Input: part model. Units: mm. Frame: model coordinates. Coordinates: 2 decimals unless noted, no trailing zeros. Write each loop counter-clockwise with the first axis right and the second up, starting at its lowest first coordinate (ties: lowest second). Pieces come first, ordered by that corner, then holes. Notation, with made-up numbers: (25.5, 31.25) - (30.5, 31.25) arc R18 ccw to (30.5, 45.25) - close; hole circle Ø9 at (5, 71.25). An arc over 180 degrees is marked (long way). Use a Markdown table: item, result. Add a question column.
Q1. Section query D-D (y = -0.75). Return the cut outline in (x, z).
Q2. Pin query (flat end, axial travel): P1, Ø1, axis at x = -9.5, z = -4, coming from the -Y side; P2, Ø2, axis at y = 5.5, z = -4, coming from the +X side; P3, Ø1.5, axis at x = 1.5, z = -3, coming from the +Y side. Return the tip coordinate at first contact, or that it passes through.
Q3. Material intervals for probe 1 along Z at (x, y) = (-10, 1); probe 2 along Y at (x, z) = (28, -3.25); probe 3 along X at (y, z) = (6, 1.75), sorted ascending. Write a range as from..to.
Q4. Section query B-B (x = -30). Return the cut outline in (y, z), then the cut area to 3 significant figures.
Q5. Section query A-A (z = -2.25). Return the cut outline in (x, y).
Autodesk Fusion 360 part; units mm, degrees
sketch "Sketch1" plane through (0, 0, 0) normal (0, 0, 1) x (1, 0, 0) in component "Cover"
  line L0 (34, 8.25) -> (-34, 8.25)
  line L1 (-34, 8.25) -> (-34, -8.25)
  line L2 (-34, -8.25) -> (34, -8.25)
  line L3 (34, -8.25) -> (34, 8.25)
  line L4 (34, 8.25) -> (-34, -8.25) construction
  line L5 (-34, 8.25) -> (34, -8.25) construction
  line L6 (-32.5, -6.75) -> (32.5, -6.75) construction
  line L7 (32.5, -6.75) -> (32.5, 6.75) construction
  line L8 (32.5, 6.75) -> (-32.5, 6.75)
  line L9 (-32.5, 6.75) -> (-32.5, -6.75) construction
  line L10 (32.5, 4.25) -> (24.6, 4.25)
  line L11 (24.6, 4.25) -> (24.6, 6.75)
  line L12 (24.6, 6.75) -> (32.5, 6.75)
  line L13 (32.5, 6.75) -> (32.5, 4.25)
  line L14 (22.9833, 6.75) -> (22.9833, 4.25)
  line L15 (15.0833, 4.25) -> (15.0833, 6.75)
  line L16 (22.9833, 4.25) -> (15.0833, 4.25)
  line L17 (15.0833, 6.75) -> (22.9833, 6.75)
  line L18 (13.4667, 6.75) -> (13.4667, 4.25)
  line L19 (5.5667, 4.25) -> (5.5667, 6.75)
  line L20 (13.4667, 4.25) -> (5.5667, 4.25)
  line L21 (5.5667, 6.75) -> (13.4667, 6.75)
  line L22 (3.95, 6.75) -> (3.95, 4.25)
  line L23 (-3.95, 4.25) -> (-3.95, 6.75)
  line L24 (3.95, 4.25) -> (-3.95, 4.25)
  line L25 (-3.95, 6.75) -> (3.95, 6.75)
  line L26 (-5.5667, 6.75) -> (-5.5667, 4.25)
  line L27 (-13.4667, 4.25) -> (-13.4667, 6.75)
  line L28 (-5.5667, 4.25) -> (-13.4667, 4.25)
  line L29 (-13.4667, 6.75) -> (-5.5667, 6.75)
  line L30 (-15.0833, 6.75) -> (-15.0833, 4.25)
  line L31 (-22.9833, 4.25) -> (-22.9833, 6.75)
  line L32 (-15.0833, 4.25) -> (-22.9833, 4.25)
  line L33 (-22.9833, 6.75) -> (-15.0833, 6.75)
  line L34 (-24.6, 6.75) -> (-24.6, 4.25)
  line L35 (-32.5, 4.25) -> (-32.5, 6.75)
  line L36 (-24.6, 4.25) -> (-32.5, 4.25)
  line L37 (-32.5, 6.75) -> (-24.6, 6.75)
  line L38 (-34, -8.25) -> (-36, -8.25)
  line L39 (-36, -8.25) -> (-36, 8.25)
  line L40 (-36, 8.25) -> (-34, 8.25)
  line L41 (-34, 8.25) -> (-34, -8.25)
  line L42 (34, -8.25) -> (36, -8.25)
  line L43 (36, -8.25) -> (36, 8.25)
  line L44 (36, 8.25) -> (34, 8.25)
  line L45 (34, 8.25) -> (34, -8.25)
  dimension "d39" = 68
  dimension "d40" = 16.5
  dimension "d42" = 7.9
  dimension "d43" = 2.5
  dimension "d46" = -57.1
  dimension "d47" = 0
  dimension "d52" = 2
  dimension "d53" = 2
extrude "Extrude1" add sketch "Sketch1" along normal blind 2 contours L0 L1 L2 L3 L41 L45 | L3 L42 L43 L44 L45 | L1 L38 L39 L40 L41 | L8 L10 L11 L12 L13 | L8 L34 L35 L36 L37 | L8 L30 L31 L32 L33 | L8 L26 L27 L28 L29 | L8 L22 L23 L24 L25 | L8 L18 L19 L20 L21 | L8 L14 L15 L16 L17 in component "Cover"
extrude "Extrude3" add sketch "Sketch1" against normal blind 5 contours L8 L10 L11 L12 L13 | L8 L34 L35 L36 L37 | L8 L30 L31 L32 L33 | L8 L26 L27 L28 L29 | L8 L22 L23 L24 L25 | L8 L18 L19 L20 L21 | L8 L14 L15 L16 L17 in component "Cover"
fillet "Fillet1" radius 3 7 edges at (28.55, 4.25, 0) (19.0333, 4.25, 0) (9.5167, 4.25, 0) (0, 4.25, 0) (-9.5167, 4.25, 0) (-19.0333, 4.25, 0) (-28.55, 4.25, 0) in component "Cover"
chamfer "Chamfer2" distance 0.4 angle 45 1 faces at (1.3167, -3.25, 2) in component "Cover"
component "Cover" placed x (1, 0, 0) y (0, 1, 0) z (0, 0, 1) at (0, 0, 0)
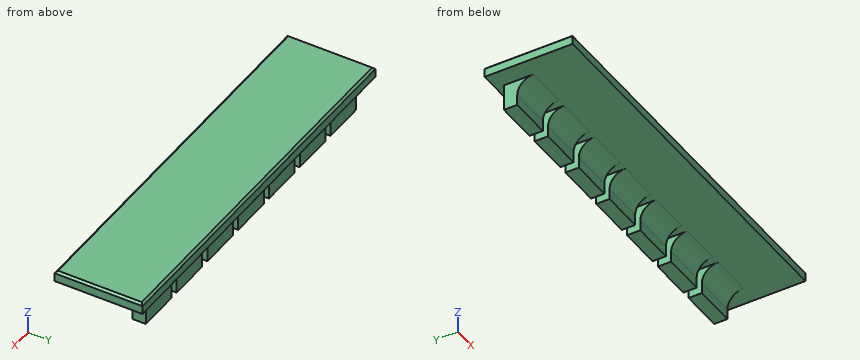
Values follow:
| question | item | result |
|---|---|---|
| 1 | outline | (-36, 0) - (36, 0) - (36, 1.6) - (35.6, 2) - (-35.6, 2) - (-36, 1.6) - close |
| 2 | P1 | y = 4.25 |
| 2 | P2 | x = 32.5 |
| 2 | P3 | y = 6.75 |
| 3 | probe 1 | 0..2 |
| 3 | probe 2 | 4.25..6.75 |
| 3 | probe 3 | -35.85..35.85 |
| 4 | outline | (-8.25, 0) - (1.25, 0) arc R3 cw to (4.25, -3) - (4.25, -5) - (6.75, -5) - (6.75, 0) - (8.25, 0) - (8.25, 1.6) - (7.85, 2) - (-7.85, 2) - (-8.25, 1.6) - close |
| 4 | area | 47.3 mm2 |
| 5 | outline | (-32.5, 4.15) - (-24.6, 4.15) - (-24.6, 6.75) - (-32.5, 6.75) - close; (-22.98, 4.15) - (-15.08, 4.15) - (-15.08, 6.75) - (-22.98, 6.75) - close; (-13.47, 4.15) - (-5.57, 4.15) - (-5.57, 6.75) - (-13.47, 6.75) - close; (-3.95, 4.15) - (3.95, 4.15) - (3.95, 6.75) - (-3.95, 6.75) - close; (5.57, 4.15) - (13.47, 4.15) - (13.47, 6.75) - (5.57, 6.75) - close; (15.08, 4.15) - (22.98, 4.15) - (22.98, 6.75) - (15.08, 6.75) - close; (24.6, 4.15) - (32.5, 4.15) - (32.5, 6.75) - (24.6, 6.75) - close |
